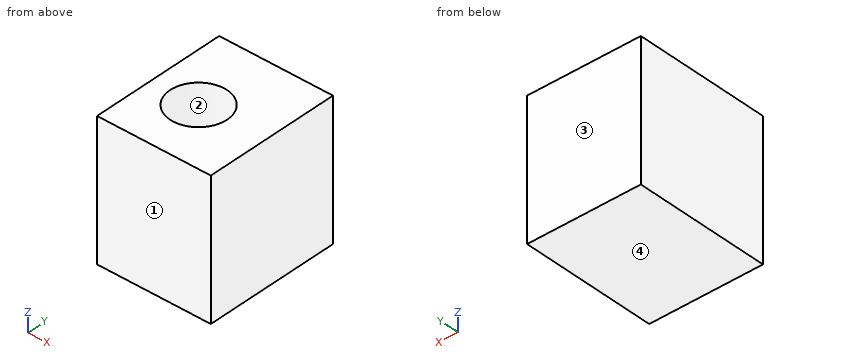
from build123d import *

# Parameters (mm, degrees)
F0_W     = 50
F0_H     = 60
F1_DEPTH = 35
F2_W     = 50
F2_H     = 60
F2_R     = 12.5
F3_DEPTH = 25
F4_R     = 15
F5_DEPTH = 30


with BuildPart() as f1:
    # F0 (on Top) → F1 (new body)
    with BuildSketch(Plane.XY):
        with Locations((25, 30)):
            Rectangle(F0_W, F0_H)
    extrude(amount=F1_DEPTH)

    # F2 (on face) → F3 (join)
    with BuildSketch(Plane.XY.offset(35)):
        with Locations((25, 30)):
            Rectangle(F2_W, F2_H)
        with Locations((20.667605, 26.786247)):
            Circle(F2_R, mode=Mode.SUBTRACT)
    extrude(amount=F3_DEPTH)

    # F4 (on face) → F5 (join)
    with BuildSketch(Plane(origin=(0, 0, 0), x_dir=(0, -1, 0), z_dir=(-1, 0, 0))):
        with Locations((-29.429901, 20.344391)):
            Circle(F4_R)
    extrude(amount=-F5_DEPTH)


solid = f1.part
Geometry: final body of the model. Coordinates: model frame, mm. Face numbers are marked on the shaded views. Give positions to 0.01 mm unless a question says otherwise; leave off trailing zeros. Loops run counter-clockwise (first coordinate to the right, second up) from the corner with the lowest first, then second, coordinate; pieces in that order, holes last. Notation, with made-up numbers: (11.25, 74) - (56.25, 74) arc R33 cw to (56.25, 110) - close; hole circle Ø9 at (57, -13). An arc over 180 degrees is marked (long way). Answer as CSV lines item,"result". Start each with the question number.
1. Section B-B, the plane x = 12. Return loops of the section in (y, z), plus the area to 3 significant figures.
2. Draft query along Y for the marked faces 1, 2, 3 and 4. Return one class per face: released by +Y, released by -Y, zero draft, split by the parting line, or undercut.
3. Section D-D, the plane x = 27.5. Return loops of the section in (y, z).
4. Ray query, L1, parallel to Y at x = 21, z = 43.5; L2, parallel to X at y = 27, z = 35.5; L3, parallel to Z at x = 21, y = 36.5. Return the intervals inside material, ascending.
5. Section C-C, the plane y = 16. Return loops of the section in (x, z).
6. Section A-A, the plane z = 48. Return loops of the section in (x, y).
7. Pin query (flat end, axial travel): P1, Ø7.5, axis at x = 15.5, y = 28.5, coming from the +Z side. Return the tip coordinate at first contact, or that it passes through.
Answers:
1,outline,"(0, 0) - (60, 0) - (60, 60) - (35.79, 60) - (35.79, 35) - (32.63, 35) arc R15 ccw to (26.23, 35) - (17.78, 35) - (17.78, 60) - (0, 60) - close"
1,area,"3,150 mm2"
2,face 1,"released by -Y"
2,face 2,"undercut"
2,face 3,"released by +Y"
2,face 4,"zero draft"
3,outline,"(0, 0) - (60, 0) - (60, 60) - (37.25, 60) - (37.25, 35) - (32.63, 35) arc R15 ccw to (26.23, 35) - (16.32, 35) - (16.32, 60) - (0, 60) - close"
4,L1,"y = 0 to 14.29, 39.28 to 60"
4,L2,"x = 0 to 8.17, 33.17 to 50"
4,L3,"z = 0 to 35"
5,outline,"(0, 0) - (50, 0) - (50, 60) - (26.98, 60) - (26.98, 35) - (14.35, 35) - (14.35, 60) - (0, 60) - close"
6,outline,"(0, 0) - (50, 0) - (50, 60) - (0, 60) - close; hole circle Ø25 at (20.67, 26.79)"
7,P1,"stops at z = 35.34"
